Part model, mm, in its own coordinate system. Face numbers are marked on the shaded views. A direction names the side the tool comes from. Coordinates: 2 decimals unless noted, no trailing zeros. Order: outer loops, then holes, each group sorted by start corner. A loop starts at its lowest first (then second) coordinate and runs counter-clockwise, first axis right, second up.
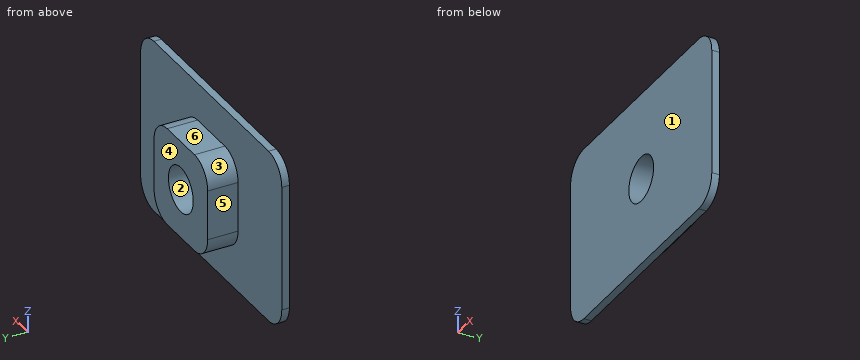
from build123d import *

# Parameters (mm, degrees)
CROQUIS1_W              = 85.5
CROQUIS1_H              = 57.5
SALIENTE_EXTRUIR1_DEPTH = 2.5
REDONDEO1_R             = 8
CROQUIS2_W              = 32.5
CROQUIS2_H              = 32.5
SALIENTE_EXTRUIR2_DEPTH = 10
REDONDEO2_R             = 8
CROQUIS3_R              = 7.5
CORTAR_EXTRUIR1_DEPTH   = 54.012970111


with BuildPart() as part:
    # Croquis1 → Saliente-Extruir1 (new body)
    with BuildSketch(Plane(origin=(0, 0, 0), x_dir=(1, 0, 0), z_dir=(0, 1, 0))):
        Rectangle(CROQUIS1_W, CROQUIS1_H)
    extrude(amount=SALIENTE_EXTRUIR1_DEPTH)

    # Redondeo1
    redondeo1_edges = [part.edges().sort_by_distance(p)[0] for p in [
        (42.75, 1.25, 28.75),
        (-42.75, 1.25, 28.75),
        (-42.75, 1.25, -28.75),
        (42.75, 1.25, -28.75),
    ]]
    fillet(redondeo1_edges, radius=REDONDEO1_R)

    # Croquis2 → Saliente-Extruir2 (add)
    with BuildSketch(Plane(origin=(0, 2.5, 0), x_dir=(1, 0, 0), z_dir=(0, 1, 0))):
        Rectangle(CROQUIS2_W, CROQUIS2_H)
    extrude(amount=SALIENTE_EXTRUIR2_DEPTH)

    # Redondeo2
    redondeo2_edges = [part.edges().sort_by_distance(p)[0] for p in [
        (16.25, 7.5, 16.25),
        (16.25, 7.5, -16.25),
        (-16.25, 7.5, -16.25),
        (-16.25, 7.5, 16.25),
    ]]
    fillet(redondeo2_edges, radius=REDONDEO2_R)

    # Croquis3 → Cortar-Extruir1 (cut, through all)
    with BuildSketch(Plane(origin=(0, 12.5, 0), x_dir=(1, 0, 0), z_dir=(0, 1, 0))):
        with Locations(Location((0, 0, 0), (0, 0, 270))):
            Circle(CROQUIS3_R)
    extrude(amount=-CORTAR_EXTRUIR1_DEPTH, mode=Mode.SUBTRACT)


solid = part.part
Q1. Which spindle directions (+Z, -Z, +X, -X, +Y, -Y) get a long thin tool onto all of the face, cutting with end or side? Do the marked faces 4, 5 and 6. Say none if no direction does.
Results list:
face 4: +Z, -Z, +X, -X, +Y
face 5: +Z, -Z, -X, +Y
face 6: +Z, +X, -X, +Y
Q2. Pin check, flat tips, straight feed: pin 1 Ø4 at (y, z) = (9, 15.5) entering from +X; pin 2 Ø3 at (y, z) = (7.5, -1.5) entering from +X; pin 3 Ø5 at (y, z) = (9.5, -3.5) entering from -X. Stop position of each tip, or through.
Results list:
pin 1: stops at x = 14.29
pin 2: stops at x = 16.25
pin 3: stops at x = -16.25
Q3. Mould opens along X. For the marked faces 1, 2 and 3 say: pulls with the +X half, pulls with the -X half, needs draft (parallel to the pull), parting line crosses it, or undercut.
Results list:
face 1: needs draft
face 2: undercut
face 3: pulls with the -X half
Q4. Wall check: line 1 along X through (y, z) = (4.25, 0); line 2 along Y through (x, z) = (-25.5, -19); line 3 along X through (y, z) = (11.5, 8.5). Give the ranges that are in metal, low to high.
Results list:
line 1: x = -16.25 to -7.5, 7.5 to 16.25
line 2: y = 0 to 2.5
line 3: x = -16.25 to 16.25
Q5. Cut at A-A on x = 0. Write the cut outline in (y, z), and give its area (3 significant figures).
Results list:
outline: (0, -28.75) - (2.5, -28.75) - (2.5, -16.25) - (12.5, -16.25) - (12.5, -7.5) - (0, -7.5) - close; (0, 7.5) - (12.5, 7.5) - (12.5, 16.25) - (2.5, 16.25) - (2.5, 28.75) - (0, 28.75) - close
area: 281 mm2
Q6. Cut at D-D on y = 1.25. Write the cut outline in (x, z).
Results list:
outline: (-42.75, -20.75) arc R8 ccw to (-34.75, -28.75) - (34.75, -28.75) arc R8 ccw to (42.75, -20.75) - (42.75, 20.75) arc R8 ccw to (34.75, 28.75) - (-34.75, 28.75) arc R8 ccw to (-42.75, 20.75) - close; hole circle Ø15 at (0, 0)
Q7. Cut at B-B on y = 9.75. Write the cut outline in (x, z), and give its area (3 significant figures).
Results list:
outline: (-16.25, -8.25) arc R8 ccw to (-8.25, -16.25) - (8.25, -16.25) arc R8 ccw to (16.25, -8.25) - (16.25, 8.25) arc R8 ccw to (8.25, 16.25) - (-8.25, 16.25) arc R8 ccw to (-16.25, 8.25) - close; hole circle Ø15 at (0, 0)
area: 825 mm2
Q8. Cut at C-C on z = 0. Write the cut outline in (x, y).
Results list:
outline: (-42.75, 0) - (-7.5, 0) - (-7.5, 12.5) - (-16.25, 12.5) - (-16.25, 2.5) - (-42.75, 2.5) - close; (7.5, 0) - (42.75, 0) - (42.75, 2.5) - (16.25, 2.5) - (16.25, 12.5) - (7.5, 12.5) - close
